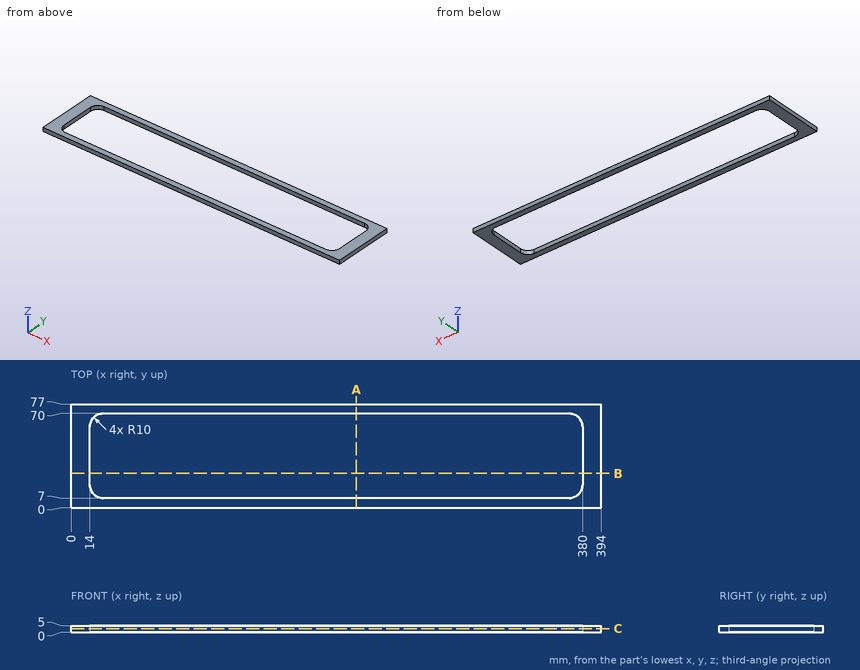
Study the drawing (mm; zero at the part's minimum x, y, z) and answer. Round coordinates to 2 decimals unless told otherwise and drop trailing zeros. Write each loop counter-clockwise with the first axis right and the second up, starting at its lowest first coordinate (ties: lowest second). Pieces come first, ordered by that corner, then holes.
1) A cutting plane is placed at C-C on z = 2.75. Determine the outline of the cut face in (x, y).
2) A cutting plane is placed at B-B on y = 25.5. Determine the outline of the cut face in (x, z).
3) Consider probe 1 along X at (y, z) = (21, 3.55); probe 2 along Y at (x, z) = (123, 2.5); probe 3 along X at (y, z) = (15.5, 4.75). Determine where each line is inside the solid, lowest interval first.
4) A cutting plane is placed at A-A on x = 212. Determine the outline of the cut face in (y, z), and give its area (3 significant figures).
Entries:
1. outline: (0, 0) - (394, 0) - (394, 77) - (0, 77) - close; hole (14, 17) arc R10 ccw to (24, 7) - (370, 7) arc R10 ccw to (380, 17) - (380, 60) arc R10 ccw to (370, 70) - (24, 70) arc R10 ccw to (14, 60) - close
2. outline: (0, 0) - (14, 0) - (14, 5) - (0, 5) - close; (380, 0) - (394, 0) - (394, 5) - (380, 5) - close
3. probe 1: x = 0 to 14, 380 to 394
3. probe 2: y = 0 to 7, 70 to 77
3. probe 3: x = 0 to 14.11, 379.89 to 394
4. outline: (0, 0) - (7, 0) - (7, 5) - (0, 5) - close; (70, 0) - (77, 0) - (77, 5) - (70, 5) - close
4. area: 70.0 mm2
